Autodesk Inventor part; units mm, degrees
ref_plane "YZ Plane" through (0, 0, 0) normal (1, 0, 0) x (0, 1, 0)
ref_plane "XZ Plane" through (0, 0, 0) normal (0, 1, 0) x (-1, 0, 0)
ref_plane "XY Plane" through (0, 0, 0) normal (0, 0, 1) x (1, 0, 0)
sketch "Sketch1" plane through (0, 0, 0) normal (0, 1, 0) x (-1, 0, 0)
  line L0 (0, 0) -> (0, -7)
  line L1 (0, -7) -> (2.5, -7)
  line L2 (2.5, -7) -> (2.5, -2.5)
  line L3 (2.5, -2.5) -> (7, -2.5)
  line L4 (7, -2.5) -> (7, 0)
  line L5 (7, 0) -> (0, 0)
  line L6 (0, -30) -> (0, -23)
  line L7 (0, -23) -> (2.5, -23)
  line L8 (2.5, -23) -> (2.5, -27.5)
  line L9 (2.5, -27.5) -> (7, -27.5)
  line L10 (7, -27.5) -> (7, -30)
  line L11 (7, -30) -> (0, -30)
  line L12 (23, 0) -> (30, 0)
  line L13 (30, 0) -> (30, -7)
  line L14 (30, -7) -> (27.5, -7)
  line L15 (27.5, -7) -> (27.5, -2.5)
  line L16 (27.5, -2.5) -> (23, -2.5)
  line L17 (23, -2.5) -> (23, 0)
  line L18 (30, -23) -> (30, -30)
  line L19 (30, -30) -> (23, -30)
  line L20 (23, -30) -> (23, -27.5)
  line L21 (23, -27.5) -> (27.5, -27.5)
  line L22 (27.5, -27.5) -> (27.5, -23)
  line L23 (27.5, -23) -> (30, -23)
  dimension "d0" = 7
  dimension "d1" = 2.5
  dimension "d2" = 4.5
  dimension "d3" = 4.5
  dimension "d8" = 7
  dimension "d9" = 4.5
  dimension "d10" = 7
  dimension "d11" = 7
  dimension "d12" = 2.5
  dimension "d13" = 30
  dimension "d14" = 30
  dimension "d15" = 30
  dimension "d16" = 2.5
  dimension "d17" = 2.5
  dimension "d18" = 4.5
  dimension "d19" = 7
extrude "Extrusion1" add sketch "Sketch1" along normal blind 20
sketch "Sketch2" plane through (0, 0, 0) normal (0, -1, 0) x (1, 0, 0)
  line L0 (0, 0) -> (-30, 0)
  line L1 (-30, 0) -> (-30, -30)
  line L2 (-30, -30) -> (0, -30)
  line L3 (0, -30) -> (0, 0)
  line L4 (-27.5, -2.5) -> (-2.5, -2.5)
  line L5 (-2.5, -2.5) -> (-2.5, -27.5)
  line L6 (-2.5, -27.5) -> (-27.5, -27.5)
  line L7 (-27.5, -27.5) -> (-23, -27.5)
  line L8 (-27.5, -27.5) -> (-27.5, -2.5)
extrude "Extrusion2" add sketch "Sketch2" against normal blind 7
sketch "Sketch3" plane through (0, 20, 0) normal (0, 1, 0) x (1, 0, 0)
  line L0 (0, 0) -> (-7, 0)
  line L1 (0, 0) -> (-30, 0)
  line L2 (-7, 0) -> (-7, 7)
  line L3 (-7, 7) -> (0, 7)
  line L4 (0, 7) -> (0, 0)
  line L5 (0, 30) -> (-7, 30)
  line L6 (-7, 30) -> (-7, 23)
  line L7 (-7, 23) -> (0, 23)
  line L8 (-2.5, 23) -> (0, 23)
  line L9 (0, 23) -> (0, 30)
  line L10 (0, 23) -> (0, 30)
  line L11 (-30, 30) -> (-30, 23)
  line L12 (-30, 0) -> (-30, 30)
  line L13 (-30, 23) -> (-23, 23)
  line L14 (-23, 23) -> (-23, 30)
  line L15 (-23, 30) -> (-30, 30)
  line L16 (-30, 30) -> (0, 30)
  line L17 (-30, 0) -> (-23, 0)
  line L18 (-23, 0) -> (-23, 7)
  line L19 (-23, 7) -> (-30, 7)
  line L20 (-27.5, 7) -> (-30, 7)
  line L21 (-30, 7) -> (-30, 0)
  dimension "d24" = 7
  dimension "d25" = 7
  dimension "d26" = 7
  dimension "d27" = 7
  dimension "d28" = 7
extrude "Extrusion3" add sketch "Sketch3" along normal blind 1
sketch "Sketch4" plane through (0, 0, 0) normal (1, 0, 0) x (0, 0, -1)
  line L0 (0, 0) -> (7, 0)
  line L1 (27.5, 0) -> (2.5, 0)
  line L2 (7, 0) -> (7, 2)
  line L3 (7, 2) -> (0, 2)
  line L4 (0, 2) -> (0, 0)
  line L5 (30, 0) -> (30, 2)
  line L6 (30, 0) -> (30, 21)
  line L7 (30, 2) -> (23, 2)
  line L8 (23, 2) -> (23, 0)
  line L9 (0, 0) -> (30, 0)
  line L10 (23, 0) -> (30, 0)
  dimension "d31" = 7
  dimension "d32" = 2
  dimension "d33" = 2
  dimension "d34" = 7
sketch "Sketch5" plane through (0, 0, -30) normal (0, 0, -1) x (-1, 0, 0)
  line L0 (0, 0) -> (7, 0)
  line L1 (7, 0) -> (7, 2)
  line L2 (7, 2) -> (0, 2)
  line L3 (0, 2) -> (0, 0)
  line L4 (30, 0) -> (30, 2)
  line L5 (30, 0) -> (30, 21)
  line L6 (30, 2) -> (23, 2)
  line L7 (23, 2) -> (23, 0)
  line L8 (23, 0) -> (30, 0)
  line L9 (30, 0) -> (0, 0)
  dimension "d35" = 7
  dimension "d36" = 2
  dimension "d37" = 2
  dimension "d38" = 7
extrude "Extrusion4" add sketch "Sketch4" along normal blind 7
extrude "Extrusion5" add sketch "Sketch5" along normal blind 7
sketch "Sketch6" plane through (0, 2, 0) normal (0, 1, 0) x (1, 0, 0)
  circle A0 centre (3.5, 3.5) radius 2
  line L0 (7, 7) -> (7, 0)
  line L1 (0, 0) -> (7, 0)
  point P0 (7, 3.5)
  point P1 (3.5, 0)
  dimension "d43" = 4
sketch "Sketch7" plane through (0, 2, -23) normal (0, 1, 0) x (1, 0, 0)
  circle A0 centre (3.5, 3.5) radius 2
  line L0 (7, 7) -> (7, 0)
  line L1 (0, 0) -> (7, 0)
  point P0 (0, -23)
  point P1 (7, 3.5)
  point P2 (3.5, 0)
  dimension "d44" = 4
sketch "Sketch8" plane through (-7, 2, -30) normal (0, 1, 0) x (1, 0, 0)
  circle A0 centre (3.5, 3.5) radius 2
  circle A1 centre (-19.5, 3.5) radius 2
  line L0 (7, 0) -> (7, 7)
  line L1 (7, 0) -> (0, 0)
  line L2 (-23, 0) -> (-23, 7)
  line L3 (-23, 7) -> (-16, 7)
  point P0 (7, -30)
  point P1 (7, 3.5)
  point P2 (3.5, 0)
  point P3 (-23, 3.5)
  point P4 (-19.5, 7)
  dimension "d45" = 4
  dimension "d46" = 4
extrude "Extrusion6" cut sketch "Sketch6" against normal blind 2
extrude "Extrusion7" cut sketch "Sketch7" against normal blind 2
extrude "Extrusion8" cut sketch "Sketch8" against normal blind 2
sketch "Sketch9" plane through (0, 21, 0) normal (0, 1, 0) x (1, 0, 0)
  line L0 (0, 30) -> (0, 0)
  line L1 (0, 0) -> (-30, 0)
  line L2 (7, 0) -> (-30, 0)
  line L3 (-30, 0) -> (-30, 30)
  line L4 (-30, 0) -> (-30, 37)
  line L5 (0, 30) -> (-30, 30)
  line L6 (-2.5, 27.5) -> (-27.5, 27.5)
  line L7 (-2.5, 27.5) -> (-27.5, 27.5)
  line L8 (-27.5, 27.5) -> (-27.5, 2.5)
  line L9 (-27.5, 2.5) -> (-2.5, 2.5)
  line L10 (-27.5, 2.5) -> (-2.5, 2.5)
  line L11 (-2.5, 2.5) -> (-2.5, 27.5)
extrude "Extrusion9" add sketch "Sketch9" against normal blind 7
sketch "Sketch10" plane through (-30, 0, 0) normal (-1, 0, 0) x (0, 0, 1)
  line L0 (0, 0) -> (-11.5, 0)
  line L1 (-2.5, 0) -> (-27.5, 0)
  line L2 (-11.5, 0) -> (-11.5, -7)
  line L3 (-11.5, -7) -> (-18.5, -7)
  line L4 (-18.5, -7) -> (-18.5, 0)
  line L5 (-18.5, 0) -> (-18.5, 7)
  line L6 (-23, 7) -> (-7, 7)
  line L7 (-18.5, 7) -> (-11.5, 7)
  line L8 (-11.5, 0) -> (-11.5, 7)
  dimension "d55" = 11.5
  dimension "d56" = 7
  dimension "d57" = 7
  dimension "d58" = 7
extrude "Extrusion10" add sketch "Sketch10" along normal blind 2
sketch "Sketch11" plane through (-30, 21, 0) normal (0, 0, 1) x (1, 0, 0)
  line L0 (0, -21) -> (11.5, -21)
  line L1 (7, -21) -> (23, -21)
  line L2 (11.5, -21) -> (18.5, -21)
  line L3 (18.5, -21) -> (18.5, -14)
  line L4 (7, -14) -> (23, -14)
  line L5 (18.5, -14) -> (11.5, -14)
  line L6 (11.5, -21) -> (11.5, -14)
  line L7 (11.5, -21) -> (11.5, -28)
  line L8 (11.5, -28) -> (18.5, -28)
  line L9 (18.5, -28) -> (18.5, -21)
  point P0 (30, -21)
  dimension "d61" = 11.5
  dimension "d62" = 7
  dimension "d63" = 7
extrude "Extrusion11" add sketch "Sketch11" along normal blind 2
sketch "Sketch12" plane through (-30, 21, 2) normal (0, 0, 1) x (1, 0, 0)
  circle A0 centre (15, -24.5) radius 2
  line L0 (18.5, -28) -> (18.5, -21)
  line L1 (11.5, -28) -> (18.5, -28)
  point P0 (30, -21)
  point P1 (18.5, -24.5)
  point P2 (15, -28)
  dimension "d66" = 4
sketch "Sketch13" plane through (-32, 0, 0) normal (-1, 0, 0) x (0, 0, 1)
  circle A0 centre (-15, -3.5) radius 2
  line L0 (-11.5, -7) -> (-11.5, 0)
  line L1 (-18.5, -7) -> (-11.5, -7)
  point P0 (0, 0)
  point P1 (-11.5, -3.5)
  point P2 (-15, -7)
  dimension "d67" = 4
extrude "Extrusion12" cut sketch "Sketch13" against normal blind 2
extrude "Extrusion13" cut sketch "Sketch12" against normal blind 2
properties part number "ygolki" material "Nylon, molybdenum disulphide"
Source: CAD feature listing. Evaluate the final solid. Frame: model axes, mm. A direction names the side the tool comes from. Round coordinates to 2 decimals unless told otherwise and drop trailing zeros. Loops run counter-clockwise (first coordinate to the right, second up) from the corner with the lowest first, then second, coordinate; pieces in that order, holes last. Notation, with made-up numbers: M 81.25,57.25 L 118.25,57.25 A20 ccw 118.25,85.25 Z; hole C -30.75,41.5 d6. An arc over 180 degrees is marked long. Return JSON: item names as keys, results as strings. Group by question number.
1. Mould query, pull axis Z, two halves, no side actions, for faces 1 (the face through (7, 1, -26)), 2 (the face through (3, 1, -30)), 3 (the face through (-16, 15, 0)), 4 (the face through (-4.7, 20.5, -23)). Classes: released by +Z, released by -Z, zero draft, split by the parting line, or undercut.
2. Section query A-A on x = -15. Output: boundary loops of the cut face in (y, z).
3. Material intervals for line 1 along X through (y, z) = (1.2, -3.5); line 2 along X through (y, z) = (1.45, -33.5); line 3 along Z through (x, y) = (-3.5, 1.1), sorted ascending. Write a range as from..to.
4. Section query C-C on y = -3.5. Output: boundary loops of the cut face in (x, z).
5. Pin query (flat end, axial travel): pin 1 (1.2 mm diameter, centred on x = -29, z = -11.5, fed in from -Y); pin 2 (10.5 mm diameter, centred on x = -16.5, y = 7, fed in from -Z); pin 3 (1.2 mm diameter, centred on x = -29, y = 10, fed in from +Z). Return the tip coordinate at first contact, or that it passes through.
6. Reachability of faces 5 (the face through (-31, 0, -11.5)), 6 (the face through (-5, 20, -25)), 7 (the face through (-1, 10, -23)), 8 (the face through (-7, 1, -33)) from +Z, -Z, +X, -X, +Y, -Y: full face, straight path, thin tool, end or side. Return the list, or none.
7. Section query D-D on x = -8.5. Output: boundary loops of the cut face in (y, z).
8. Section query B-B on z = -3.5. Output: boundary loops of the cut face in (x, y), and give its area (3 significant figures).
Checks:
{
 "1": {"face 1": "zero draft", "face 2": "released by -Z", "face 3": "released by +Z", "face 4": "undercut"},
 "2": {"outline": "M -7,0 L -5.5,0 L -5.5,2 L -7,2 Z; M -1.5,0 L 0,0 L 0,-2.5 L 7,-2.5 L 7,2 L -1.5,2 Z; M 0,-30 L 7,-30 L 7,-27.5 L 0,-27.5 Z; M 14,-30 L 21,-30 L 21,-27.5 L 14,-27.5 Z; M 14,-2.5 L 21,-2.5 L 21,0 L 14,0 Z"},
 "3": {"line 1": "x = -30..-27.5, -2.5..1.5, 5.5..7", "line 2": "x = -30..-28.5, -24.5..-23, -7..-5.5, -1.5..0", "line 3": "z = -37..-35.5, -31.5..-27.5, -2.5..0"},
 "4": {"outline": "M -32,-18.5 L -30,-18.5 L -30,-17 L -32,-17 Z; M -32,-13 L -30,-13 L -30,-11.5 L -32,-11.5 Z; M -18.5,0 L -17,0 L -17,2 L -18.5,2 Z; M -13,0 L -11.5,0 L -11.5,2 L -13,2 Z"},
 "5": {"pin 1": "stops at y = 0", "pin 2": "stops at z = -30", "pin 3": "stops at z = 0"},
 "6": {"face 5": "+Z, -X, +Y, -Y", "face 6": "-Y", "face 7": "+X, -X", "face 8": "-Z, +Y, -Y"},
 "7": {"outline": "M 0,-30 L 7,-30 L 7,-27.5 L 0,-27.5 Z; M 0,-2.5 L 7,-2.5 L 7,0 L 0,0 Z; M 14,-30 L 21,-30 L 21,-27.5 L 14,-27.5 Z; M 14,-2.5 L 21,-2.5 L 21,0 L 14,0 Z"},
 "8": {"outline": "M -30,0 L -27.5,0 L -27.5,20 L -23,20 L -23,21 L -30,21 Z; M -7,20 L -2.5,20 L -2.5,0 L 1.5,0 L 1.5,2 L 0,2 L 0,21 L -7,21 Z; M 5.5,0 L 7,0 L 7,2 L 5.5,2 Z", "area": "120 mm²"}
}
